Study the drawing (mm; zero at the part's minimum x, y, z) and answer. Round coordinates to 2 decimals unless told otherwise and drop trailing zeros. Order: outer loops, then holes, each group sorted by start corner. A loop starts at its lowest first (then second) coordinate and runs counter-clockwise, first axis right, second up. Notation, with made-up numbers: (75, -31) -> (89, -31) arc R28 ccw to (89, 8) -> close; hole circle Ø1 at (18.25, 56). An arc over 180 degrees is marked (long way). Answer in a Markdown table with one row per item. Add a question column.
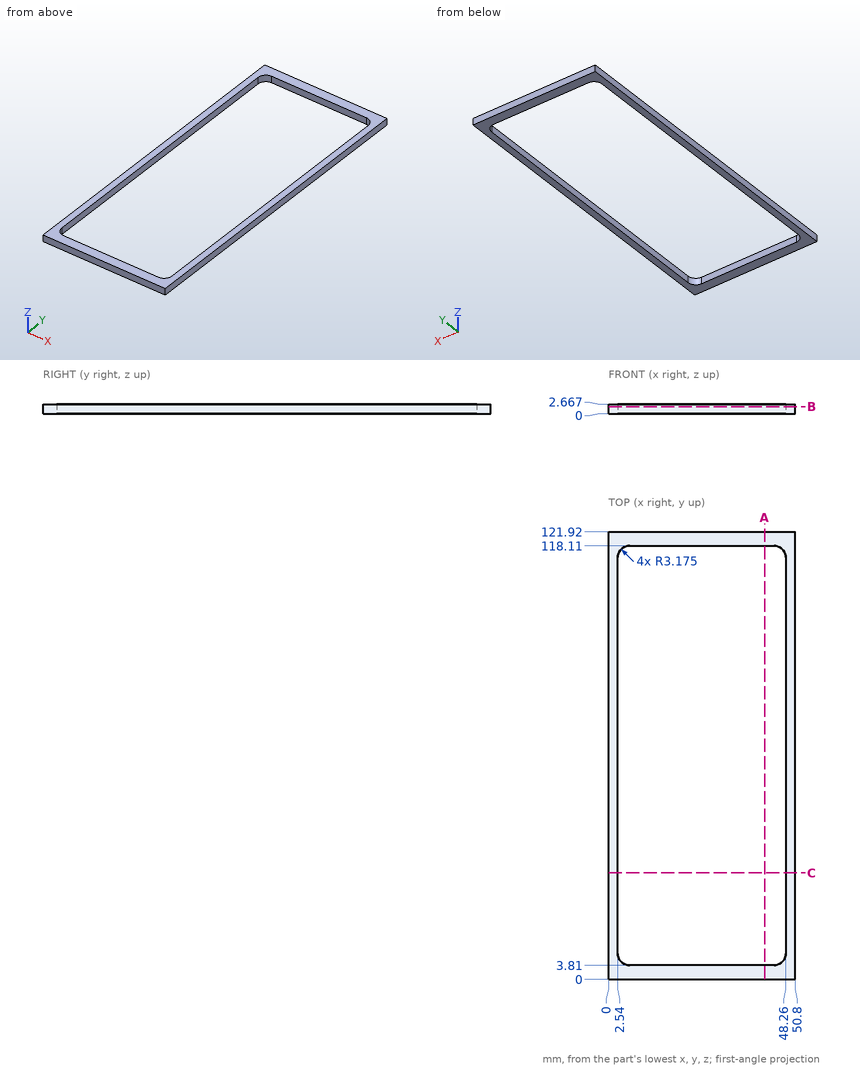
Item 1: The part is cut by section C-C, the plane y = 29. Give the vertices of the cut face in (x, z), and give its area (3 significant figures).
Item 2: The part is cut by section A-A, the plane x = 42.5. Give the vertices of the cut face in (y, z), and give its area (3 significant figures).
Item 3: The part is cut by section B-B, the plane z = 1.95. Give the vertices of the cut face in (x, y) (3 decimals).
Item 4: Find the intervals of material crossed by probe 1 along X at (y, z) = (32.5, 2); probe 2 along Y at (x, z) = (30.5, 1.1); probe 3 along Y at (x, z) = (3.5, 2), in increasing order. Write a range as [from, to].
Resolved:
| question | item | result |
|---|---|---|
| 1 | outline | (0, 0) -> (2.54, 0) -> (2.54, 2.67) -> (0, 2.67) -> close; (48.26, 0) -> (50.8, 0) -> (50.8, 2.67) -> (48.26, 2.67) -> close |
| 1 | area | 13.5 mm2 |
| 2 | outline | (0, 0) -> (3.81, 0) -> (3.81, 2.67) -> (0, 2.67) -> close; (118.11, 0) -> (121.92, 0) -> (121.92, 2.67) -> (118.11, 2.67) -> close |
| 2 | area | 20.3 mm2 |
| 3 | outline | (0, 0) -> (50.8, 0) -> (50.8, 121.92) -> (0, 121.92) -> close; hole (2.54, 6.985) arc R3.175 ccw to (5.715, 3.81) -> (45.085, 3.81) arc R3.175 ccw to (48.26, 6.985) -> (48.26, 114.935) arc R3.175 ccw to (45.085, 118.11) -> (5.715, 118.11) arc R3.175 ccw to (2.54, 114.935) -> close |
| 4 | probe 1 | [0, 2.54], [48.26, 50.8] |
| 4 | probe 2 | [0, 3.81], [118.11, 121.92] |
| 4 | probe 3 | [0, 4.71], [117.21, 121.92] |
